Work out the finished part from the listing and answer in its coordinate system (mm). Round coordinates to 2 decimals unless told otherwise and drop trailing zeros. Order: outer loops, then holes, each group sorted by start corner. A loop starts at its lowest first (then second) coordinate and runs counter-clockwise, first axis right, second up. Notation, with made-up numbers: (-9.5, 17) - (35.5, 17) arc R18 cw to (35.5, 38) - close; hole circle Ø8 at (-20.75, 27.25). An arc over 180 degrees is marked (long way). One line per question, with ' | ' between items. Start each with the question number.
Autodesk Inventor part; units mm, degrees
ref_plane "YZ Plane" through (0, 0, 0) normal (1, 0, 0) x (0, 1, 0)
ref_plane "XZ Plane" through (0, 0, 0) normal (0, 1, 0) x (-1, 0, 0)
ref_plane "XY Plane" through (0, 0, 0) normal (0, 0, 1) x (1, 0, 0)
sketch "Sketch1" plane through (0, 0, 0) normal (0, 1, 0) x (-1, 0, 0)
  line L0 (0, 0) -> (-42.0116, 0)
  line L1 (-42.0116, 0) -> (-42.0116, -228.6)
  line L2 (-42.0116, -228.6) -> (0, -228.6)
  line L3 (0, -228.6) -> (0, 0)
  circle A0 centre (-21.0058, -12.7) radius 3.175
  circle A1 centre (-21.0058, -215.9) radius 3.175
  circle A2 centre (-3.048, -28.448) radius 2.0193
  circle A3 centre (-38.9636, -64.3636) radius 2.0193
  line L4 (0, 0) -> (101.6, 12.7)
  line L5 (101.6, 12.7) -> (177.8, 12.7)
  line L6 (304.8, -114.3) -> (304.8, -114.3)
  line L7 (177.8, -241.3) -> (101.6, -241.3)
  line L8 (101.6, -241.3) -> (0, -228.6)
  circle A4 centre (177.8, -114.3) radius 76.2
  arc A5 (304.8, -114.3) -> (177.8, 12.7) centre (177.8, -114.3) ccw
  arc A6 (177.8, -241.3) -> (304.8, -114.3) centre (177.8, -114.3) ccw
  point P0 (304.8, 12.7)
  point P1 (304.8, -241.3)
  dimension "d0" = 42.0116
  dimension "d1" = 228.6
  dimension "d2" = 12.7
  dimension "d3" = 12.7
  dimension "d4" = 6.35
  dimension "d5" = 21.0058
  dimension "d6" = 21.0058
  dimension "d7" = 6.35
  dimension "d8" = 28.448
  dimension "d9" = 3.048
  dimension "d10" = 4.0386
  dimension "d11" = 4.0386
  dimension "d12" = 64.3636
  dimension "d13" = 3.048
  dimension "d21" = 152.4
  dimension "d22" = 254
  dimension "d23" = 203.2
  dimension "d24" = 101.6
  dimension "d25" = 127
  dimension "d26" = 127
  dimension "d27" = 127
  dimension "d28" = 127
extrude "Extrusion1" add sketch "Sketch1" along normal blind 3.175
sketch "Sketch2" plane through (0, 3.175, 0) normal (0, 1, 0) x (1, 0, 0)
  circle A0 centre (21.0058, 46.4058) radius 7.9375
  line L0 (0, 228.6) -> (0, 0)
  line L1 (0, 0) -> (42.0116, 0)
  line L2 (42.0116, 228.6) -> (0, 228.6)
  line L3 (0, 0) -> (0, 228.6)
  line L4 (42.0116, 0) -> (42.0116, 228.6)
  dimension "d16" = 15.875
  dimension "d18" = 46.4058
  dimension "d31" = 21.0058
extrude "Extrusion2" cut sketch "Sketch2" against normal blind 7.9375 contours A0
fillet "Fillet1" radius 152.4 2 edges at (-101.6, 1.5875, 12.7) (-101.6, 1.5875, -241.3)
sketch "Sketch3" plane through (0, 3.175, 0) normal (0, 1, 0) x (1, 0, 0)
  circle A0 centre (-177.8, 114.3) radius 107.95 construction
  circle A1 centre (-177.8, 114.3) radius 76.2
  circle A2 centre (-177.8, 6.35) radius 2.5781
  circle A3 centre (-69.85, 114.3) radius 2.5781
  circle A4 centre (-177.8, 222.25) radius 2.5781
  circle A5 centre (-285.75, 114.3) radius 2.5781
  line L0 (-177.8, 114.3) -> (-177.8, 6.35) construction
  line L1 (-177.8, 114.3) -> (-69.85, 114.3) construction
  line L2 (-177.8, 114.3) -> (-177.8, 222.25) construction
  line L3 (-177.8, 114.3) -> (-285.75, 114.3) construction
  point P0 (0, 0)
  dimension "d33" = 215.9
  dimension "d35" = 90
  dimension "d43" = 90
  dimension "d44" = 90
extrude "Extrusion3" cut sketch "Sketch3" against normal blind 25.4 contours A2 | A3 | A4 | A5
properties part number "BAG motor top plate" material "Aluminum 6061"
1) Determine the mould class of faces 1 (the flat face through (-46.738, 1.565, -234.442)), 2 (the flat face through (-90, 3.175, -113)), 3 (the cylindrical face through (24.668, 1.61, -39.364)), 4 (the cylindrical face through (-117.33, 1.565, -67.933)) for opening direction X: released by +X, released by -X, zero draft, split by the parting line, or undercut.
2) Straight lines are drawn through the part: line 1 (Z direction, x = -177.8, y = 1.55); line 2 (X direction, y = 2.5, z = -6.35); line 3 (Z direction, x = -138, y = 2.5). For each, find the intervals that lie inside material, in ascending order.
3) Section A-A on z = -79.5 is taken. Give the vertices of the cut face in (x, y) (3 decimals).
4) Section D-D on x = -12.5 is taken. Give the vertices of the cut face in (y, z) (1 decimal).
5) Flat-ended cylindrical pins translate along their axes: pin 1 (3 mm diameter, centred on x = 38.96, z = -64.36, fed in from +Y) (3 decimals); pin 2 (1 mm diameter, centred on x = 12.5, y = 2.5, fed in from +Z). Find the tip coordinate at first contact, or state that the pin passes through.
6) Section C-C on y = 1.4 is taken. Give the number of separate pieces and of enclosed holes in the cut face, and give its area (3 significant figures).
7) Section B-B on x = -197.5 is taken. Give the vertices of the cut face in (y, z) (3 decimals), and give its area (3 significant figures).
Recorded:
1) face 1: released by +X | face 2: zero draft | face 3: undercut | face 4: undercut
2) line 1: z = -241.3 to -224.83, -219.67 to -190.5, -38.1 to -8.93, -3.77 to 12.7 | line 2: x = -244.7 to -180.38, -175.22 to 42.01 | line 3: z = -241.3 to -179.28, -49.32 to 12.7
3) outline: (-299.939, 0) - (-245.589, 0) - (-245.589, 3.175) - (-299.939, 3.175) - close; (-110.011, 0) - (42.012, 0) - (42.012, 3.175) - (-110.011, 3.175) - close
4) outline: (0, -230.2) - (3.2, -230.2) - (3.2, 1.6) - (0, 1.6) - close
5) pin 1: passes through | pin 2: stops at z = 0
6) separate pieces: 1 | enclosed holes: 10 | area: 60,200 mm²
7) outline: (0, -239.763) - (3.175, -239.763) - (3.175, -187.909) - (0, -187.909) - close; (0, -40.691) - (3.175, -40.691) - (3.175, 11.163) - (0, 11.163) - close | area: 329 mm²
